Geometry check sheet. Reference: the model listing, model coordinates, mm. A direction names the side the tool comes from. Coordinates: 2 decimals unless noted, no trailing zeros. Write each loop counter-clockwise with the first axis right and the second up, starting at its lowest first coordinate (ties: lowest second). Pieces come first, ordered by that corner, then holes. Notation, with made-up numbers: (-13.5, -35.5) -> (5.5, -35.5) arc R21 cw to (5.5, -29.5) -> close; hole circle Ø3 at (-21, 26). An arc over 180 degrees is marked (long way). Answer as CSV lines item,"result".
```python
from build123d import *

# Parameters (mm, degrees)
BOSS_EXTRUDE1_DEPTH        = 8
CUT_EXTRUDE1_DEPTH         = 283.696502476
F_6_5_6_5_DIAMETER_HOLE2_D = 6.5


with BuildPart() as part:
    # Sketch1 → Boss-Extrude1 (new body)
    with BuildSketch(Plane.XY.offset(8)):
        Polygon((-154.499999959, -218.249999957), (154.500000044, -218.249999957), (179.500000086, -193.249999916), (179.500000086, 193.249999916), (154.500000044, 218.249999957), (-154.499999959, 218.249999957), (-179.5, 193.249999916), (-179.5, -193.249999916), align=None)
    extrude(amount=-BOSS_EXTRUDE1_DEPTH)

    # Sketch2 → Cut-Extrude1 (cut, through all)
    with BuildSketch(Plane(origin=(0, 0, 0), x_dir=(-1, 0, 0), z_dir=(0, 0, -1))):
        with BuildLine():
            Line((-107.857864329, -153.249999987), (107.857864423, -153.249999987))
            ThreePointArc((107.857864423, -153.249999987), (111.684698748, -152.488795312), (114.928932237, -150.321067798))
            Line((114.928932237, -150.321067798), (129.071067861, -136.178932174))
            ThreePointArc((129.071067861, -136.178932174), (131.23879537, -132.934698692), (132.000000044, -129.107864376))
            Line((132.000000044, -129.107864376), (132.000000044, 129.107864376))
            ThreePointArc((132.000000044, 129.107864376), (131.23879537, 132.934698692), (129.071067861, 136.178932174))
            Line((129.071067861, 136.178932174), (114.928932237, 150.321067798))
            ThreePointArc((114.928932237, 150.321067798), (111.684698748, 152.488795312), (107.857864423, 153.249999987))
            Line((107.857864423, 153.249999987), (-107.857864329, 153.249999987))
            ThreePointArc((-107.857864329, 153.249999987), (-111.684698653, 152.488795312), (-114.928932143, 150.321067798))
            Line((-114.928932143, 150.321067798), (-129.071067767, 136.178932174))
            ThreePointArc((-129.071067767, 136.178932174), (-131.238795276, 132.934698692), (-131.999999949, 129.107864376))
            Line((-131.999999949, 129.107864376), (-131.999999949, -129.107864376))
            ThreePointArc((-131.999999949, -129.107864376), (-131.238795276, -132.934698692), (-129.071067767, -136.178932174))
            Line((-129.071067767, -136.178932174), (-114.928932143, -150.321067798))
            ThreePointArc((-114.928932143, -150.321067798), (-111.684698653, -152.488795312), (-107.857864329, -153.249999987))
        make_face()
    extrude(amount=-CUT_EXTRUDE1_DEPTH, mode=Mode.SUBTRACT)

    # Ø6.5 (6.5) Diameter Hole2 (through all)
    with Locations(Plane(origin=(0, 0, 0), x_dir=(-1, 0, 0), z_dir=(0, 0, -1))):
        with Locations((-153.5, -182.25), (153.5, -182.25), (-153.5, 182.25), (153.5, 182.25)):
            Hole(F_6_5_6_5_DIAMETER_HOLE2_D / 2)


solid = part.part
```
Item 1: Cross-section at C-C, the plane x = 95. Record the cut outline in (y, z), plus the area to 3 significant figures.
Responses:
outline,"(-218.25, 0) -> (-153.25, 0) -> (-153.25, 8) -> (-218.25, 8) -> close; (153.25, 0) -> (218.25, 0) -> (218.25, 8) -> (153.25, 8) -> close"
area,"1,040 mm2"
Item 2: Set-up check for faces 1 (the flat face through (122.1, -143.15, 3.94)), 2 (the flat face through (-166.825, 205.925, 4.056)): record each of +Z, -Z, +X, -X, +Y, -Y from which the full face is reachable in a straight line by a thin tool's end or side.
Responses:
face 1,"+Z, -Z"
face 2,"+Z, -Z, -X, +Y"
Item 3: Release check for a two-part mould opening along X. For faces 3 (the flat face through (166.83, -205.92, 4.06)), 4 (the flat face through (121.9, 143.35, 3.94)), 5 (the flat face through (-167.175, -205.575, 4.056)) record: +X half, -X half, draft (parallel to the pull), parting line (faces both ways), or undercut.
Responses:
face 3,"+X half"
face 4,"undercut"
face 5,"-X half"
Item 4: Cross-section at A-A, the plane y = -17.5. Record the cut outline in (x, z).
Responses:
outline,"(-179.5, 0) -> (-132, 0) -> (-132, 8) -> (-179.5, 8) -> close; (132, 0) -> (179.5, 0) -> (179.5, 8) -> (132, 8) -> close"
Item 5: Cross-section at B-B, the plane z = 4.25. Record the cut outline in (x, y), plus the area to 3 significant figures.
Responses:
outline,"(-179.5, -193.25) -> (-154.5, -218.25) -> (154.5, -218.25) -> (179.5, -193.25) -> (179.5, 193.25) -> (154.5, 218.25) -> (-154.5, 218.25) -> (-179.5, 193.25) -> close; hole circle Ø6.5 at (-153.5, -182.25); hole circle Ø6.5 at (-153.5, 182.25); hole (-132, -129.11) arc R10 ccw to (-129.07, -136.18) -> (-114.93, -150.32) arc R10 ccw to (-107.86, -153.25) -> (107.86, -153.25) arc R10 ccw to (114.93, -150.32) -> (129.07, -136.18) arc R10 ccw to (132, -129.11) -> (132, 129.11) arc R10 ccw to (129.07, 136.18) -> (114.93, 150.32) arc R10 ccw to (107.86, 153.25) -> (-107.86, 153.25) arc R10 ccw to (-114.93, 150.32) -> (-129.07, 136.18) arc R10 ccw to (-132, 129.11) -> close; hole circle Ø6.5 at (153.5, -182.25); hole circle Ø6.5 at (153.5, 182.25)"
area,"75,200 mm2"
Item 6: Thickness scan on probe 1 along X at (y, z) = (182.25, 2.5); probe 2 along Y at (x, z) = (31.5, 2); probe 3 along Y at (x, z) = (-153.5, 4). Record the ranges inside material, lowest first.
Responses:
probe 1,"x = -179.5 to -156.75, -150.25 to 150.25, 156.75 to 179.5"
probe 2,"y = -218.25 to -153.25, 153.25 to 218.25"
probe 3,"y = -218.25 to -185.5, -179 to 179, 185.5 to 218.25"
